Read the model definition and answer for the solid it produces. Units are mm, in the model's axes. Coordinates: 2 decimals unless noted, no trailing zeros. Loops run counter-clockwise (first coordinate to the right, second up) from the corner with the lowest first, then second, coordinate; pieces in that order, holes last.
Q1. Section B-B (y = 68.5) is taken. Give the vertices of the cut face in (x, z).
Q2. Straight lines are drawn through the part: line 1 (X direction, y = 42, z = 0.3); line 2 (X direction, y = 57, z = 1.3); line 3 (Y direction, x = -21.5, z = 1.1). For each, find the intervals that lie inside material, in ascending order.
Q3. Section C-C (y = 91.5) is taken. Give the vertices of the cut face in (x, z).
Q4. A flat-ended cylindrical pin translates along its axis: P1, Ø2, axis at x = -28.44, y = 38.01, coming from the -Z side. Find the tip coordinate at first contact, or state that the pin passes through.
Q5. Section A-A (z = 2.55) is taken. Give the vertices of the cut face in (x, y), then the cut area to 3 significant figures.
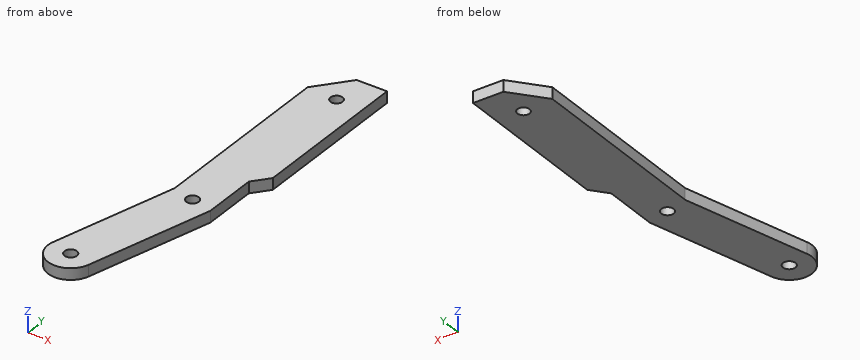
from build123d import *

# Parameters (mm, degrees)
SKETCH1_R           = 1.65
SKETCH1_R_2         = 1.6
BOSS_EXTRUDE1_DEPTH = 3


with BuildPart() as part:
    # Sketch1 → Boss-Extrude1 (new body)
    with BuildSketch(Plane.XY):
        with BuildLine():
            Line((-43.203651579, 6.54376887), (-34.230867434, 39.585145796))
            Line((-34.230867434, 39.585145796), (-34.230867434, 89.585145796))
            Line((-34.230867434, 89.585145796), (-27.230867434, 98.07042717))
            Line((-27.230867434, 98.07042717), (-19.230867434, 98.07042717))
            Line((-19.230867434, 98.07042717), (-19.230867434, 55.070526621))
            Line((-19.230867434, 55.070526621), (-22.650283011, 50.925569007))
            Line((-22.650283011, 50.925569007), (-22.650283011, 36.440298517))
            Line((-22.650283011, 36.440298517), (-31.623067155, 3.398921591))
            ThreePointArc((-31.623067155, 3.398921591), (-38.985783006, -0.818946981), (-43.203651579, 6.54376887))
        make_face()
        with Locations((-28.440575223, 38.012722157)):
            Circle(SKETCH1_R, mode=Mode.SUBTRACT)
        with Locations((-37.413359367, 4.97134523)):
            Circle(SKETCH1_R, mode=Mode.SUBTRACT)
        with Locations((-26.230867434, 89.07042717)):
            Circle(SKETCH1_R_2, mode=Mode.SUBTRACT)
    extrude(amount=BOSS_EXTRUDE1_DEPTH)


solid = part.part
Numbers:
1. outline: (-34.23, 0) - (-19.23, 0) - (-19.23, 3) - (-34.23, 3) - close
2. line 1: x = -34.23 to -22.65
2. line 2: x = -34.23 to -19.23
2. line 3: y = 52.32 to 98.07
3. outline: (-32.65, 0) - (-19.23, 0) - (-19.23, 3) - (-32.65, 3) - close
4. P1: passes through
5. outline: (-43.2, 6.54) arc R6 ccw to (-31.62, 3.4) - (-22.65, 36.44) - (-22.65, 50.93) - (-19.23, 55.07) - (-19.23, 98.07) - (-27.23, 98.07) - (-34.23, 89.59) - (-34.23, 39.59) - close; hole circle Ø3.3 at (-37.41, 4.97); hole circle Ø3.3 at (-28.44, 38.01); hole circle Ø3.2 at (-26.23, 89.07)
5. area: 1,260 mm2
